Can you work these out from the model? Positions are in its coordinate system, mm. A direction names the side the tool comes from. Coordinates: 2 decimals unless noted, no trailing zeros. Order: outer loops, then holes, each group sorted by start corner. A loop starts at its lowest first (then second) coordinate and runs counter-clockwise, first axis right, second up. Notation, with made-up numbers: (44.25, -20) -> (70.25, -20) arc R8 ccw to (70.25, -7) -> close; hole circle Ø8 at (50.25, -20.75). An arc over 180 degrees is marked (long way). Answer as CSV lines item,"result".
from build123d import *

# Parameters (mm, degrees)
SKETCH1_R           = 4.05
SKETCH1_R_2         = 1.55
SKETCH1_R_3         = 2
SKETCH1_R_4         = 3
SKETCH1_W           = 9
SKETCH1_H           = 15
BOSS_EXTRUDE1_DEPTH = 5
CUT_EXTRUDE1_DEPTH  = 6
SKETCH3_R           = 1.5
CUT_EXTRUDE2_DEPTH  = 6
CUT_EXTRUDE4_DEPTH  = 6
CIRPATTERN1_COUNT   = 3


with BuildPart() as part:
    # Sketch1 → Boss-Extrude1 (new body)
    with BuildSketch(Plane.XY):
        with BuildLine():
            Line((-127.025, 27.9715045), (39.288466521, 123.992629166))
            Line((39.288466521, 123.992629166), (37.788477193, 126.590686893))
            ThreePointArc((37.788477193, 126.590686893), (43.313466521, 128.071103321), (48.838455849, 126.590686893))
            Line((48.838455849, 126.590686893), (85.211522807, 105.590686893))
            ThreePointArc((85.211522807, 105.590686893), (89.256095707, 101.546113993), (90.736512135, 96.021124665))
            Line((90.736512135, 96.021124665), (87.736533479, 96.021124665))
            Line((87.736533479, 96.021124665), (87.736533479, -96.021124665))
            Line((87.736533479, -96.021124665), (90.736512135, -96.021124665))
            ThreePointArc((90.736512135, -96.021124665), (89.394693991, -101.298780185), (85.695118183, -105.29468591))
            Line((85.695118183, -105.29468591), (48.841497032, -126.58893042))
            ThreePointArc((48.841497032, -126.58893042), (43.315221896, -128.071103182), (37.788476129, -126.590686279))
            Line((37.788476129, -126.590686279), (39.288465746, -123.992628719))
            Line((39.288465746, -123.992628719), (-127.024990103, -27.971485569))
            Line((-127.024990103, -27.971485569), (-128.524990392, -30.569561613))
            ThreePointArc((-128.524990392, -30.569561613), (-132.569562534, -26.524988796), (-134.049978656, -21))
            Line((-134.049978656, -21), (-134.049978656, 21))
            ThreePointArc((-134.049978656, 21), (-132.569562227, 26.524989328), (-128.524989328, 30.569562227))
            Line((-128.524989328, 30.569562227), (-127.025, 27.9715045))
        make_face()
        with Locations((-123, 21)):
            Circle(SKETCH1_R, mode=Mode.SUBTRACT)
        with Locations((-123, -21)):
            Circle(SKETCH1_R, mode=Mode.SUBTRACT)
        with Locations((43.313466521, 117.021124665)):
            Circle(SKETCH1_R, mode=Mode.SUBTRACT)
        with Locations((79.686533479, 96.021124665)):
            Circle(SKETCH1_R, mode=Mode.SUBTRACT)
        with Locations((79.686533479, -96.021124665)):
            Circle(SKETCH1_R, mode=Mode.SUBTRACT)
        with Locations((43.313466521, -117.021124665)):
            Circle(SKETCH1_R, mode=Mode.SUBTRACT)
        with Locations((-110.5, 21)):
            Circle(SKETCH1_R_2, mode=Mode.SUBTRACT)
        with Locations((-110.5, -21)):
            Circle(SKETCH1_R_2, mode=Mode.SUBTRACT)
        with Locations((73.436533479, 85.195807118)):
            Circle(SKETCH1_R_2, mode=Mode.SUBTRACT)
        with Locations((37.063466521, 106.195807118)):
            Circle(SKETCH1_R_2, mode=Mode.SUBTRACT)
        with Locations((37.063466521, -106.195807118)):
            Circle(SKETCH1_R_2, mode=Mode.SUBTRACT)
        with Locations((73.436533479, -85.195807118)):
            Circle(SKETCH1_R_2, mode=Mode.SUBTRACT)
        Circle(SKETCH1_R_3, mode=Mode.SUBTRACT)
        with Locations((-92, 0)):
            Circle(SKETCH1_R_4, mode=Mode.SUBTRACT)
        with Locations((46, 79.674337148)):
            Circle(SKETCH1_R_4, mode=Mode.SUBTRACT)
        with Locations((46, -79.674337148)):
            Circle(SKETCH1_R_4, mode=Mode.SUBTRACT)
        Polygon((70.245190528, 106.668238983), (65.745190528, 98.874010348), (52.754809472, 106.374010348), (57.254809472, 114.168238983), align=None, mode=Mode.SUBTRACT)
        with Locations((-123, 0)):
            Rectangle(SKETCH1_W, SKETCH1_H, mode=Mode.SUBTRACT)
        Polygon((57.254809472, -114.168238983), (52.754809472, -106.374010348), (65.745190528, -98.874010348), (70.245190528, -106.668238983), align=None, mode=Mode.SUBTRACT)
    extrude(amount=BOSS_EXTRUDE1_DEPTH)

    # Sketch2 → Cut-Extrude1 (cut, through all)
    with BuildSketch(Plane.XY.offset(5)):
        Polygon((87.736533479, 1.48), (78.736533479, 1.48), (78.736533479, 3.5), (78.236533479, 3.5), (78.236533479, 2.75), (75.736533479, 2.75), (75.736533479, 1.48), (73.736533479, 1.48), (73.736533479, -1.48), (75.736533479, -1.48), (75.736533479, -2.75), (78.236533479, -2.75), (78.236533479, -3.5), (78.736533479, -3.5), (78.736533479, -1.48), (87.736533479, -1.48), align=None)
        Polygon((-43.236068195, -77.847066833), (-38.736068195, -70.052838199), (-36.986696879, -71.062838199), (-36.736696879, -70.629825497), (-37.386215932, -70.254825497), (-36.136215932, -68.089761988), (-37.236068195, -67.454761988), (-36.236068195, -65.72271118), (-38.79950339, -64.24271118), (-39.79950339, -65.974761988), (-40.899355653, -65.339761988), (-42.149355653, -67.504825497), (-42.798874706, -67.129825497), (-43.048874706, -67.562838199), (-41.29950339, -68.572838199), (-45.79950339, -76.367066833), align=None)
        Polygon((-46.449022443, 75.242066833), (-41.949022443, 67.447838199), (-43.698393759, 66.437838199), (-43.448393759, 66.004825497), (-42.798874706, 66.379825497), (-41.548874706, 64.214761988), (-40.449022443, 64.849761988), (-39.449022443, 63.11771118), (-36.885587248, 64.59771118), (-37.885587248, 66.329761988), (-36.785734985, 66.964761988), (-38.035734985, 69.129825497), (-37.386215932, 69.504825497), (-37.636215932, 69.937838199), (-39.385587248, 68.927838199), (-43.885587248, 76.722066833), align=None)
    extrude(amount=-CUT_EXTRUDE1_DEPTH, mode=Mode.SUBTRACT)

    # Sketch3 → Cut-Extrude2 (cut, through all)
    with BuildSketch(Plane.XY.offset(5)):
        with Locations((-81.705432956, -49.517948353)):
            Circle(SKETCH3_R)
        with Locations((-2.03110092, -95.517957208)):
            Circle(SKETCH3_R)
        with Locations((55.468910149, 4.074957836)):
            Circle(SKETCH3_R)
        with Locations((-24.205421887, 50.074966692)):
            Circle(SKETCH3_R)
        with BuildLine():
            Line((-112.802559279, -37.337512553), (-100.678204404, -44.337513901))
            ThreePointArc((-100.678204404, -44.337513901), (-99.91938537, -44.437414408), (-99.31217896, -43.971488649))
            Line((-99.31217896, -43.971488649), (-93.812177901, -34.445209818))
            ThreePointArc((-93.812177901, -34.445209818), (-93.712277394, -33.686390784), (-94.178203153, -33.079184374))
            Line((-94.178203153, -33.079184374), (-106.302558028, -26.079183026))
            ThreePointArc((-106.302558028, -26.079183026), (-107.061377062, -25.97928252), (-107.668583473, -26.445208278))
            Line((-107.668583473, -26.445208278), (-113.168584531, -35.971487109))
            ThreePointArc((-113.168584531, -35.971487109), (-113.268485038, -36.730306143), (-112.802559279, -37.337512553))
        make_face()
        with BuildLine():
            Line((25.432070618, -115.992612669), (30.932069559, -106.466332616))
            ThreePointArc((30.932069559, -106.466332616), (31.031969897, -105.70751356), (30.566044003, -105.100307253))
            Line((30.566044003, -105.100307253), (18.441687572, -98.1003086))
            ThreePointArc((18.441687572, -98.1003086), (17.682868516, -98.000408262), (17.075662209, -98.466334156))
            Line((17.075662209, -98.466334156), (11.575663268, -107.992614209))
            ThreePointArc((11.575663268, -107.992614209), (11.47576293, -108.751433265), (11.941688824, -109.358639572))
            Line((11.941688824, -109.358639572), (24.066045255, -116.358638224))
            ThreePointArc((24.066045255, -116.358638224), (24.824864311, -116.458538563), (25.432070618, -115.992612669))
        make_face()
    extrude(amount=-CUT_EXTRUDE2_DEPTH, mode=Mode.SUBTRACT)

    # Sketch6 → Cut-Extrude4 (cut, through all)
    with BuildSketch(Plane.XY.offset(5)):
        with BuildLine():
            ThreePointArc((-77.076260937, 44.5), (-82.225278394, 34.05882548), (-85.96739854, 23.034895014))
            ThreePointArc((-85.96739854, 23.034895014), (-84.553184977, 20.585405271), (-82.103695235, 21.999618834))
            ThreePointArc((-82.103695235, 21.999618834), (-78.529760263, 32.528091751), (-73.612159322, 42.5))
            ThreePointArc((-73.612159322, 42.5), (-74.344210129, 45.232050808), (-77.076260937, 44.5))
        make_face()
        with BuildLine():
            ThreePointArc((-73.612159322, -42.5), (-74.344210129, -45.232050808), (-77.076260937, -44.5))
            ThreePointArc((-77.076260937, -44.5), (-82.225278394, -34.05882548), (-85.96739854, -23.034895014))
            ThreePointArc((-85.96739854, -23.034895014), (-84.553184977, -20.585405271), (-82.103695235, -21.999618834))
            ThreePointArc((-82.103695235, -21.999618834), (-78.529760263, -32.528091751), (-73.612159322, -42.5))
        make_face()
    cut_extrude4 = extrude(amount=-CUT_EXTRUDE4_DEPTH, mode=Mode.SUBTRACT)

    # CirPattern1: Cut-Extrude4 ×3 about axis
    cirpattern1_axis = Axis((0, 0, 0), (0, 0, 1))
    for i in range(1, CIRPATTERN1_COUNT):
        add(cut_extrude4.rotate(cirpattern1_axis, i * 360 / CIRPATTERN1_COUNT), mode=Mode.SUBTRACT)


solid = part.part
Q1. Which directions (+Z, -Z, +X, -X, +Y, -Y) give clear straight access to the entire face, cutting with the end or side of a thin tool? Please do faces 1 (the cylindrical face through (-82.163, -34.209, 2.535)), 2 (the flat face through (-120, -32.027, 2.465)), 3 (the flat face through (5, 2, 5)).
Solution:
face 1,"+Z, -Z"
face 2,"+Z, -Z, -Y"
face 3,"+Z, +X, -X, +Y, -Y"
Q2. If I drill on line 1 (Y direction, x = -40, z = 1.4); line 2 (X direction, y = 24.5, z = 2.6); line 3 (Y direction, x = -125, z = 4.7), over which ranges is the centre line in solid material (lowest first)?
Solution:
line 1,"-78.22 to -72.24, -65.86 to 64.07, 69.99 to 78.22"
line 2,"-133.48 to -125.04, -120.96 to -85.56, -81.39 to 87.74"
line 3,"-29.14 to -24.52, -17.48 to -7.5, 7.5 to 17.48, 24.52 to 29.14"
Q3. For P1, Ø2.5, axis at x = 89, z = 1.5, coming from the -Y side; P2, Ø2, axis at y = -46.5, z = 4, coming from the -X side; P3, Ø0.6, axis at y = -2, z = 2.5, coming from the +X side, each with a flat end and sliding along its axis, tell me the tip position at first contact or that it passes through.
Solution:
P1,"y = -103.58"
P2,"x = -96.66"
P3,"x = 87.74"
Q4. Imagine slicing it at A-A (y = -55.5). List the corners of the cut face in (x, z) for me, and give its area (3 significant figures).
Solution:
outline,"(-79.34, 0) -> (64.38, 0) -> (64.38, 5) -> (-79.34, 5) -> close; (69.58, 0) -> (87.74, 0) -> (87.74, 5) -> (69.58, 5) -> close"
area,"809 mm2"
Q5. Imagine slicing it at C-C (z = 1.1). Give the number of separate pieces and of enclosed holes in the cut face, and give its area (3 significant figures).
Solution:
separate pieces,"1"
enclosed holes,"29"
area,"35,100 mm2"
Q6. We'd pull the mould along Y, two halves only. Please class faces 4 (the cylindrical face through (89.215, 101.616, 2.465)), 5 (the cylindrical face through (42.436, -120.975, 2.465)), 6 (the flat face through (-110.38, -31.14, 2.54)): pulls with the +Y half, pulls with the -Y half, needs draft (parallel to the pull), parting line crosses it, or undercut.
Solution:
face 4,"pulls with the +Y half"
face 5,"undercut"
face 6,"pulls with the -Y half"
Q7. Imagine slicing it at B-B (x = -8). List the corners of the cut face in (y, z) for me.
Solution:
outline,"(-96.69, 0) -> (96.69, 0) -> (96.69, 5) -> (-96.69, 5) -> close"
